Work out the finished part from the listing and answer in its coordinate system (mm). A direction names the side the tool comes from. Give positions to 0.01 mm unless a question says otherwise; leave off trailing zeros. Loops run counter-clockwise (first coordinate to the right, second up) from the corner with the lowest first, then second, coordinate; pieces in that order, holes last. Notation, with made-up numbers: M -17,76.5 L 4,76.5 A15 cw 4,93.5 Z; hole C 22,5 d3. An arc over 180 degrees is marked long. Use a Markdown table: item, result.
```python
from build123d import *

# Parameters (mm, degrees)
ESBO_O23_W                     = 44.3
ESBO_O23_H                     = 11.5
ESBO_O23_R                     = 2
FLANGE_BASE2_DEPTH             = 3
ARESTA_FLANGE1_STRIP_W         = 13.4732
ARESTA_FLANGE1_STRIP_H         = 3
ARESTA_FLANGE1_STRIP_CUT_DEPTH = 44.3
ARESTA_FLANGE1_DEPTH           = 44.3
CORTE_EXTRUS_O1_REACH          = 41.939
CORTE_EXTRUS_O2_REACH          = 41.939
ESBO_O33_R                     = 1.5
ESBO_O33_W                     = 10
ESBO_O33_H                     = 11.0034
FILETE1_START                  = -5
FILETE1_DEPTH                  = 12.011168151
FILETE1_START_2                = 4.011168151
FILETE1_2_DEPTH                = 3
FILETE1_3_DEPTH                = 3
FILETE1_START_3                = -4
FILETE1_4_DEPTH                = 4.7366001
ESBO_O34_W                     = 23.8
ESBO_O34_H                     = 4.7634
CORTE_EXTRUS_O3_DEPTH          = 39.884804768
FILETE2_R                      = 2


with BuildPart() as part:
    # Flange-base2: sheet metal written as solids
    # Esboço23 → Flange-base2 (new body)
    with BuildSketch(Plane(origin=(0, 0, 0), x_dir=(1, 0, 0), z_dir=(0, 1, 0))):
        with Locations((13.143114832, -1.261168151)):
            Rectangle(ESBO_O23_W, ESBO_O23_H)
        with Locations(Location((-3.756885168, 0.488831849, 0), (0, 0, 270))):
            Circle(ESBO_O23_R, mode=Mode.SUBTRACT)
        with Locations(Location((30.043114832, 0.488831849, 0), (0, 0, 90))):
            Circle(ESBO_O23_R, mode=Mode.SUBTRACT)
    extrude(amount=-FLANGE_BASE2_DEPTH)

    # Aresta-Flange1: sheet metal written as solids
    # Aresta-Flange1 strip (on a plane across the edge) → Aresta-Flange1 strip cut (cut)
    with BuildSketch(Plane(origin=(-9.006885168, 0, 7.011168151), x_dir=(0, 0, -1), z_dir=(1, 0, 0))):
        with Locations((-3, -1.5)):
            Rectangle(ARESTA_FLANGE1_STRIP_W, ARESTA_FLANGE1_STRIP_H)
    extrude(amount=ARESTA_FLANGE1_STRIP_CUT_DEPTH, mode=Mode.SUBTRACT)

    # Aresta-Flange1 section (on a plane across the edge) → Aresta-Flange1 (add)
    with BuildSketch(Plane(origin=(-9.006885168, 0, 7.011168151), x_dir=(0, 0, -1), z_dir=(1, 0, 0))):
        with BuildLine():
            Line((0, 0.7366), (0, 14.74))
            Line((0, 14.74), (3, 14.74))
            Line((3, 14.74), (3, 0.7366))
            ThreePointArc((3, 0.7366), (3.215745145, 0.215745145), (3.7366, 0))
            Line((3.7366, 0), (3.7366, -3))
            ThreePointArc((3.7366, -3), (1.094424801, -1.905575199), (0, 0.7366))
        make_face()
    extrude(amount=ARESTA_FLANGE1_DEPTH)

    # Esboço31 → Corte-extrusão1 (cut, up to next)
    with BuildSketch(Plane.XY.offset(7.011168151), mode=Mode.PRIVATE) as corte_extrus_o1_sk1:
        with BuildLine():
            Line((5.143114832, 14.74), (5.143114832, 11.99))
            Line((5.143114832, 11.99), (3.393114832, 11.99))
            ThreePointArc((3.393114832, 11.99), (0.641414832, 9.2383), (3.393114832, 6.4866))
            Line((3.393114832, 6.4866), (5.143114832, 6.4866))
            Line((5.143114832, 6.4866), (5.143114832, 0.7366))
            Line((5.143114832, 0.7366), (-9.006885168, 0.7366))
            Line((-9.006885168, 0.7366), (-9.006885168, 14.74))
            Line((-9.006885168, 14.74), (5.143114832, 14.74))
        make_face()
    corte_extrus_o1_tool1 = extrude(corte_extrus_o1_sk1.sketch, amount=-CORTE_EXTRUS_O1_REACH, mode=Mode.PRIVATE) & part.part
    # Esboço31 → Corte-extrusão1 (cut, up to next)
    with BuildSketch(Plane.XY.offset(7.011168151), mode=Mode.PRIVATE) as corte_extrus_o1_sk2:
        with BuildLine():
            Line((21.143114832, 6.4866), (21.143114832, 0.7366))
            Line((21.143114832, 0.7366), (35.293114832, 0.7366))
            Line((35.293114832, 0.7366), (35.293114832, 14.74))
            Line((35.293114832, 14.74), (21.143114832, 14.74))
            Line((21.143114832, 14.74), (21.143114832, 11.99))
            Line((21.143114832, 11.99), (22.893114832, 11.99))
            ThreePointArc((22.893114832, 11.99), (25.644814832, 9.2383), (22.893114832, 6.4866))
            Line((22.893114832, 6.4866), (21.143114832, 6.4866))
        make_face()
    corte_extrus_o1_tool2 = extrude(corte_extrus_o1_sk2.sketch, amount=-CORTE_EXTRUS_O1_REACH, mode=Mode.PRIVATE) & part.part
    add(corte_extrus_o1_tool1.solids().sort_by_distance((-2.549902, 7.555498, 7.011168))[0], mode=Mode.SUBTRACT)
    add(corte_extrus_o1_tool2.solids().sort_by_distance((28.836132, 7.555498, 7.011168))[0], mode=Mode.SUBTRACT)

    # Esboço33 → Corte-extrusão2 (cut, up to next)
    with BuildSketch(Plane.XY.offset(7.011168151), mode=Mode.PRIVATE) as corte_extrus_o2_sk1:
        with Locations((3.393114832, 9.2383)):
            Circle(ESBO_O33_R)
    corte_extrus_o2_tool1 = extrude(corte_extrus_o2_sk1.sketch, amount=-CORTE_EXTRUS_O2_REACH, mode=Mode.PRIVATE) & part.part
    # Esboço33 → Corte-extrusão2 (cut, up to next)
    with BuildSketch(Plane.XY.offset(7.011168151), mode=Mode.PRIVATE) as corte_extrus_o2_sk2:
        with Locations(Location((22.893114832, 9.2383, 0), (0, 0, 180))):
            Circle(ESBO_O33_R)
    corte_extrus_o2_tool2 = extrude(corte_extrus_o2_sk2.sketch, amount=-CORTE_EXTRUS_O2_REACH, mode=Mode.PRIVATE) & part.part
    # Esboço33 → Corte-extrusão2 (cut, up to next)
    with BuildSketch(Plane.XY.offset(7.011168151), mode=Mode.PRIVATE) as corte_extrus_o2_sk3:
        with Locations((13.143114832, 9.2383)):
            Rectangle(ESBO_O33_W, ESBO_O33_H)
    corte_extrus_o2_tool3 = extrude(corte_extrus_o2_sk3.sketch, amount=-CORTE_EXTRUS_O2_REACH, mode=Mode.PRIVATE) & part.part
    add(corte_extrus_o2_tool1.solids().sort_by_distance((3.393115, 9.2383, 7.011168))[0], mode=Mode.SUBTRACT)
    add(corte_extrus_o2_tool2.solids().sort_by_distance((22.893115, 9.2383, 7.011168))[0], mode=Mode.SUBTRACT)
    add(corte_extrus_o2_tool3.solids().sort_by_distance((13.143115, 9.2383, 7.011168))[0], mode=Mode.SUBTRACT)

    # Filete1: read off the stored shape, not the designer's step
    # Filete1 outline → Filete1 (cut)
    with BuildSketch(Plane.XY.offset(FILETE1_START)):
        with BuildLine():
            Line((-9.006885168, 0.7366), (-9.006885168, -1.2634))
            ThreePointArc((-9.006885168, -1.2634), (-8.42109873, 0.150813562), (-7.006885168, 0.7366))
            Line((-7.006885168, 0.7366), (-9.006885168, 0.7366))
        make_face()
        with BuildLine():
            ThreePointArc((33.293114832, 0.7366), (34.707328395, 0.150813562), (35.293114832, -1.2634))
            Line((35.293114832, -1.2634), (35.293114832, 0.7366))
            Line((35.293114832, 0.7366), (33.293114832, 0.7366))
        make_face()
    extrude(amount=FILETE1_DEPTH, mode=Mode.SUBTRACT)

    # Filete1 2 outline → Filete1 2 (add)
    with BuildSketch(Plane.XY.offset(FILETE1_START_2)):
        with BuildLine():
            ThreePointArc((5.143114832, 2.7366), (4.557328394, 1.322386438), (3.143114832, 0.7366))
            Line((3.143114832, 0.7366), (5.143114832, 0.7366))
            Line((5.143114832, 0.7366), (5.143114832, 2.7366))
        make_face()
        with BuildLine():
            Line((21.143114832, 0.7366), (23.143114832, 0.7366))
            ThreePointArc((23.143114832, 0.7366), (21.72890127, 1.322386438), (21.143114832, 2.7366))
            Line((21.143114832, 2.7366), (21.143114832, 0.7366))
        make_face()
        with BuildLine():
            Line((8.143114832, 3.7366), (10.143114832, 3.7366))
            ThreePointArc((10.143114832, 3.7366), (8.72890127, 4.322386438), (8.143114832, 5.7366))
            Line((8.143114832, 5.7366), (8.143114832, 3.7366))
        make_face()
        with BuildLine():
            ThreePointArc((18.143114832, 5.7366), (17.557328394, 4.322386437), (16.143114832, 3.7366))
            Line((16.143114832, 3.7366), (18.143114832, 3.7366))
            Line((18.143114832, 3.7366), (18.143114832, 5.7366))
        make_face()
    extrude(amount=FILETE1_2_DEPTH)

    # Filete1 3 outline → Filete1 3 (add)
    with BuildSketch(Plane.XY.offset(FILETE1_START_2)):
        with BuildLine():
            ThreePointArc((22.893114832, 11.99), (22.96552716, 11.989047052), (23.037889334, 11.986188868))
            ThreePointArc((23.037889334, 11.986188868), (21.69217531, 12.606910766), (21.143114832, 13.983418849))
            Line((21.143114832, 13.983418849), (21.143114832, 11.99))
            Line((21.143114832, 11.99), (22.893114832, 11.99))
        make_face()
        with BuildLine():
            ThreePointArc((21.143114832, 4.493181151), (21.69217531, 5.869689234), (23.037889334, 6.490411131))
            ThreePointArc((23.037889334, 6.490411131), (22.96552716, 6.487552948), (22.893114832, 6.4866))
            Line((22.893114832, 6.4866), (21.143114832, 6.4866))
            Line((21.143114832, 6.4866), (21.143114832, 4.493181151))
        make_face()
        with BuildLine():
            ThreePointArc((5.143114832, 13.983418849), (4.594054355, 12.606910766), (3.248340331, 11.986188869))
            ThreePointArc((3.248340331, 11.986188869), (3.320702504, 11.989047052), (3.393114832, 11.99))
            Line((3.393114832, 11.99), (5.143114832, 11.99))
            Line((5.143114832, 11.99), (5.143114832, 13.983418849))
        make_face()
        with BuildLine():
            ThreePointArc((3.248340331, 6.490411131), (4.594054355, 5.869689234), (5.143114832, 4.493181151))
            Line((5.143114832, 4.493181151), (5.143114832, 6.4866))
            Line((5.143114832, 6.4866), (3.393114832, 6.4866))
            ThreePointArc((3.393114832, 6.4866), (3.320702504, 6.487552948), (3.248340331, 6.490411131))
        make_face()
    extrude(amount=FILETE1_3_DEPTH)

    # Filete1 4 outline → Filete1 4 (cut)
    with BuildSketch(Plane(origin=(0, 0, 0), x_dir=(1, 0, 0), z_dir=(0, 1, 0)).offset(FILETE1_START_3)):
        with BuildLine():
            Line((35.293114832, 4.488831849), (33.293114832, 4.488831849))
            ThreePointArc((33.293114832, 4.488831849), (34.707328395, 3.903045412), (35.293114832, 2.488831849))
            Line((35.293114832, 2.488831849), (35.293114832, 4.488831849))
        make_face()
        with BuildLine():
            ThreePointArc((-9.006885168, 2.488831849), (-8.421098731, 3.903045412), (-7.006885168, 4.488831849))
            Line((-7.006885168, 4.488831849), (-9.006885168, 4.488831849))
            Line((-9.006885168, 4.488831849), (-9.006885168, 2.488831849))
        make_face()
    extrude(amount=FILETE1_4_DEPTH, mode=Mode.SUBTRACT)

    # Esboço34 → Corte-extrusão3 (cut, through all)
    with BuildSketch(Plane(origin=(0, 0, 0), x_dir=(1, 0, 0), z_dir=(0, 1, 0))):
        with Locations((13.143114832, 2.107131849)):
            Rectangle(ESBO_O34_W, ESBO_O34_H)
    extrude(amount=-CORTE_EXTRUS_O3_DEPTH, mode=Mode.SUBTRACT)

    # Filete2
    # the kernel refuses this fillet: 2 mm, written as the material it adds along each edge
    with BuildSketch(Plane(origin=(1.243114832, 0, 0.274568151), x_dir=(0, 0, -1), z_dir=(0, -1, 0))) as filete2_piece_1:
        with BuildLine():
            CenterArc((FILETE2_R, FILETE2_R), FILETE2_R, 180, 90)
            Line((0, FILETE2_R), (0, 0))
            Line((0, 0), (FILETE2_R, 0))
        make_face()
    extrude(amount=3)
    with BuildSketch(Plane(origin=(25.043114832, 0, 0.274568151), x_dir=(0, 0, -1), z_dir=(0, -1, 0))) as filete2_piece_2:
        with BuildLine():
            CenterArc((FILETE2_R, -FILETE2_R), FILETE2_R, 90, 90)
            Line((0, -FILETE2_R), (0, 0))
            Line((0, 0), (FILETE2_R, 0))
        make_face()
    extrude(amount=3)
    # the kernel refuses this fillet: 2 mm, written as the material it takes off along each edge
    with BuildSketch(Plane(origin=(5.143114832, 14.74, 11.515742565), x_dir=(1, 0, 0), z_dir=(0, 0, -1))) as filete2_2_piece_1:
        with BuildLine():
            CenterArc((1.801829766, 2), FILETE2_R, 198.110746947, 71.889253053)
            Line((-0.099085117, 1.378290576), (-0.289176606, 1.316119634))
            ThreePointArc((-0.289176606, 1.316119634), (-0.2, 0.756581151), (-0.2, 0))
            Line((-0.2, 0), (0, -0.2))
            Line((0, -0.2), (1.801829766, -0.2))
            Line((1.801829766, -0.2), (1.801829766, 0))
        make_face()
    extrude(amount=12.009148828, mode=Mode.SUBTRACT)
    with BuildSketch(Plane(origin=(21.143114832, 14.74, 11.515742565), x_dir=(0.07170480855584176, -0.9974258972124044, 0), z_dir=(0, 0, -1))) as filete2_2_piece_2:
        with BuildLine():
            CenterArc((1.865651936, 1.940601288), FILETE2_R, 184.111911668, 71.889253032)
            Line((-0.129199858, 1.797191671), (-0.328685038, 1.782850709))
            Line((-0.328685038, 1.782850709), (-0.199485179, -0.014340962))
            Line((-0.199485179, -0.014340962), (0.014340962, -0.199485179))
            ThreePointArc((0.014340962, -0.199485179), (0.768974595, -0.145234673), (1.333467159, -0.194060129))
            Line((1.333467159, -0.194060129), (1.381847593, 0))
        make_face()
    extrude(amount=12.009148828, mode=Mode.SUBTRACT)
    with BuildSketch(Plane(origin=(8.143114832, 14.74, 12.011168151), x_dir=(0, -1, 0), z_dir=(0, 0, -1)), Plane(origin=(18.143114832, 14.74, 12.011168151), x_dir=(1, 0, 0), z_dir=(0, 0, -1)), Plane(origin=(25.043114832, 5, -4.488831849), x_dir=(1, 0, 0), z_dir=(0, -1, 0))) as filete2_2_piece_3:
        with BuildLine():
            CenterArc((FILETE2_R, FILETE2_R), FILETE2_R, 180, 90)
            Line((0, FILETE2_R), (0, 0))
            Line((0, 0), (FILETE2_R, 0))
        make_face()
    extrude(amount=13, mode=Mode.SUBTRACT)
    with BuildSketch(Plane(origin=(1.243114832, 5, -4.488831849), x_dir=(-1, 0, 0), z_dir=(0, -1, 0))) as filete2_2_piece_4:
        with BuildLine():
            CenterArc((FILETE2_R, -FILETE2_R), FILETE2_R, 90, 90)
            Line((0, -FILETE2_R), (0, 0))
            Line((0, 0), (FILETE2_R, 0))
        make_face()
    extrude(amount=13, mode=Mode.SUBTRACT)


solid = part.part
```
(1) Consider probe 1 along X at (y, z) = (8.5, 5.25); probe 2 along X at (y, z) = (9.75, 6); probe 3 along Y at (x, z) = (22, 2.5). Determine where each line is inside the solid, lowest interval first. Write a range as [from, to].
Entries:
| item | result |
|---|---|
| probe 1 | x = [0.74, 2.09], [4.7, 8.14], [18.14, 21.59], [24.2, 25.54] |
| probe 2 | x = [0.69, 1.98], [4.8, 8.14], [18.14, 21.48], [24.3, 25.6] |
| probe 3 | y = [-3, 0] |
(2) Which of the six approach directions +Z, -Z, +X, -X, +Y, -Y give full straight-line access (tool end or side, diameter ignored) to faces 1 (the cylindrical face through (21.678, 5.854, 5.49)), 2 (the cylindrical face through (4.579, 5.885, 5.49)), 3 (the cylindrical face through (7.68, 14.02, 5.53))?
Entries:
| item | result |
|---|---|
| face 1 | +Z, -Z, +X |
| face 2 | +Z, -Z, -X |
| face 3 | +Z, -Z, +Y |
(3) A cutting plane is placed at C-C (y = -0.5). Write down the section's boundary in (x, z), and give its area (3 significant figures).
Entries:
| item | result |
|---|---|
| outline | M -8.86,-3.25 A2 ccw -7.01,-4.49 L -0.76,-4.49 A2 ccw 1.24,-2.49 L 1.24,-1.73 A2 cw 3.24,0.27 L 23.04,0.27 A2 cw 25.04,-1.73 L 25.04,-2.49 A2 ccw 27.04,-4.49 L 33.29,-4.49 A2 ccw 35.14,-3.25 L 35.14,6.8 L -8.86,6.8 Z; hole C -3.76,-0.49 d4; hole C 30.04,-0.49 d4 |
| area | 357 mm² |
(4) A cutting plane is placed at B-B (x = 31.5). Write down the section's boundary in (y, z), and give its area (3 significant figures).
Entries:
| item | result |
|---|---|
| outline | M -3,-4.49 L 0,-4.49 L 0,-1.86 L -3,-1.86 Z; M -3,0.88 L 0,0.88 L 0,3.27 A0.74 cw 0.74,4.01 L 0.74,7.01 A3.74 ccw -3,3.27 Z |
| area | 25.6 mm² |
(5) A cutting plane is placed at A-A (y = 11.25). Write down the section's boundary in (x, z).
Entries:
| item | result |
|---|---|
| outline | M 1.52,4.01 L 8.14,4.01 L 8.14,7.01 L 1.52,7.01 Z; M 18.14,4.01 L 24.77,4.01 L 24.77,7.01 L 18.14,7.01 Z |
(6) The mould has two halves that part along X. Classify faces 4 (the flat face through (13, -3, 1)), 5 (the cylindrical face through (2.288, 10.252, 5.532)), 6 (the flat face through (5.143, 4, 6)): released by +X, released by -X, zero draft, split by the parting line, or undercut.
Entries:
| item | result |
|---|---|
| face 4 | zero draft |
| face 5 | undercut |
| face 6 | released by -X |
(7) Given P1, Ø8, axis at x = -2, y = 5.5, coming from the -Z side; P2, Ø1.5, axis at x = 26, z = 5.5, coming from the +Y side; P3, Ø1.9, axis at y = 4, z = 5.5, coming from the -X side; P4, Ø3.5, axis at x = 30.04, z = -0.49, coming from the -Y side, each flat-ended and moving along its own axis, determine where each tip first touches the part or whether it passes through.
Entries:
| item | result |
|---|---|
| P1 | stops at z = 4.01 |
| P2 | stops at y = 10.66 |
| P3 | stops at x = 5.09 |
| P4 | passes through |
(8) A cutting plane is placed at D-D (z = -1). Write down the section's boundary in (x, y).
Entries:
| item | result |
|---|---|
| outline | M -9.01,-3 L -5.69,-3 L -5.69,0 L -8.56,0 A2 ccw -9.01,-1.26 Z; M -1.82,-3 L 1.38,-3 L 1.38,0 L -1.82,0 Z; M 24.91,-3 L 28.11,-3 L 28.11,0 L 24.91,0 Z; M 31.98,-3 L 35.29,-3 L 35.29,-1.26 A2 ccw 34.84,0 L 31.98,0 Z |
